```python
from build123d import *

# Parameters (mm, degrees)
SKETCH_1_W               = 30
SKETCH_1_H               = 60
EXTRUDE_1_DEPTH          = 3
SKETCH_2_W               = 26
SKETCH_2_H               = 2
EXTRUDE_3_DEPTH          = 70
SKETCH_4_R               = 5
CUT_EXTRUDE_2_DEPTH      = 21.5
CUT_EXTRUDE_3_DEPTH      = 91.58835466
CUT_EXTRUDE_3_DEPTH_BACK = 91.58835466
SKETCH_5_R               = 1.5
SKETCH_7_W               = 29.85954739
SKETCH_7_H               = 3
EXTRUDE_4_DEPTH          = 3
CUT_EXTRUDE_5_DEPTH      = 82.504601097
CUT_EXTRUDE_5_DEPTH_BACK = 82.504601097
SKETCH_8_R               = 2


with BuildPart() as part:
    # 草图1 → 凸台-拉伸1 (new body)
    with BuildSketch(Plane(origin=(0, 0, 0), x_dir=(1, 0, 0), z_dir=(0, 1, 0))):
        Rectangle(SKETCH_1_W, SKETCH_1_H)
    extrude(amount=EXTRUDE_1_DEPTH)

    # 草图2 → 凸台-拉伸3 (add)
    with BuildSketch(Plane(origin=(0, 3, 0), x_dir=(1, 0, 0), z_dir=(0, 1, 0))):
        with Locations((0, 22)):
            Rectangle(SKETCH_2_W, SKETCH_2_H)
        with Locations((0, -22)):
            Rectangle(SKETCH_2_W, SKETCH_2_H)
    extrude(amount=EXTRUDE_3_DEPTH)

    # 草图4 → 切除-拉伸2 (cut, symmetric)
    with BuildSketch(Plane.XY):
        with Locations((0, 53)):
            Circle(SKETCH_4_R)
    extrude(amount=CUT_EXTRUDE_2_DEPTH, both=True, mode=Mode.SUBTRACT)

    # 草图5 → 切除-拉伸3 (cut, two sides: drawn at the far end of the back side and taken through both)
    with BuildSketch(Plane.XY.offset(-21.5).offset(-CUT_EXTRUDE_3_DEPTH_BACK)):
        with Locations((0, 53)):
            Circle(SKETCH_5_R)
    extrude(amount=CUT_EXTRUDE_3_DEPTH + CUT_EXTRUDE_3_DEPTH_BACK, mode=Mode.SUBTRACT)

    # 草图7 → 凸台-拉伸4 (add)
    with BuildSketch(Plane.XZ):
        Polygon((-14.929773695, 33), (-14.929773695, 30), (-12, 30), (14.929773695, 30), (14.929773695, 33), align=None)
        with Locations((0, -31.5)):
            Rectangle(SKETCH_7_W, SKETCH_7_H)
    extrude(amount=-EXTRUDE_4_DEPTH)

    # 草图8 → 切除-拉伸5 (cut, two sides: drawn at the far end of the back side and taken through both)
    with BuildSketch(Plane.XZ.offset(-CUT_EXTRUDE_5_DEPTH_BACK)):
        with BuildLine():
            ThreePointArc((-8.929773695, 29), (-9.515560133, 30.414213562), (-10.929773695, 31))
            Line((-10.929773695, 31), (-10.929773695, 29))
            Line((-10.929773695, 29), (-12.929773695, 29))
            ThreePointArc((-12.929773695, 29), (-10.929773695, 27), (-8.929773695, 29))
        make_face()
        with BuildLine():
            Line((-10.929773695, 29), (-10.929773695, 31))
            ThreePointArc((-10.929773695, 31), (-12.343987258, 30.414213562), (-12.929773695, 29))
            Line((-12.929773695, 29), (-10.929773695, 29))
        make_face()
        with Locations(Location((10.929773695, 29, 0), (0, 0, 270))):
            Circle(SKETCH_8_R)
        with Locations(Location((-10.929773695, -29, 0), (0, 0, 270))):
            Circle(SKETCH_8_R)
        with Locations(Location((10.929773695, -29, 0), (0, 0, 270))):
            Circle(SKETCH_8_R)
    extrude(amount=CUT_EXTRUDE_5_DEPTH + CUT_EXTRUDE_5_DEPTH_BACK, mode=Mode.SUBTRACT)


solid = part.part
```
Can you work these out from the model? Positions are in its coordinate system, mm. A direction names the side the tool comes from. Round coordinates to 2 decimals unless told otherwise and drop trailing zeros. Order: outer loops, then holes, each group sorted by start corner. A loop starts at its lowest first (then second) coordinate and runs counter-clockwise, first axis right, second up.
(1) If we section it at B-B (x = 0): Please give me the cut outline in (y, z).
Results are:
outline: (0, -33) - (3, -33) - (3, -23) - (51.5, -23) - (51.5, -21.5) - (48, -21.5) - (48, -21) - (3, -21) - (3, 21) - (48, 21) - (48, 21.5) - (51.5, 21.5) - (51.5, 23) - (3, 23) - (3, 33) - (0, 33) - close; (54.5, -23) - (73, -23) - (73, -21) - (58, -21) - (58, -21.5) - (54.5, -21.5) - close; (54.5, 21.5) - (58, 21.5) - (58, 21) - (73, 21) - (73, 23) - (54.5, 23) - close
(2) We'd pull the mould along Z, two halves only. Please class faces 6 (the face through (0, 1, -33)), 7 (the face through (-0.325, 51.536, 22.239)), 8 (the face through (-1.2, 54.2, 21.5)): +Z half, -Z half, draft (parallel to the pull), parting line (faces both ways), or undercut.
Results are:
face 6: -Z half
face 7: draft
face 8: undercut
(3) If we section it at A-A (y = 53): Please give me the cut outline in (x, z), plus the area to 3 significant figures.
Results are:
outline: (-13, -23) - (-1.5, -23) - (-1.5, -21.5) - (-5, -21.5) - (-5, -21) - (-13, -21) - close; (-13, 21) - (-5, 21) - (-5, 21.5) - (-1.5, 21.5) - (-1.5, 23) - (-13, 23) - close; (1.5, -23) - (13, -23) - (13, -21) - (5, -21) - (5, -21.5) - (1.5, -21.5) - close; (1.5, 21.5) - (5, 21.5) - (5, 21) - (13, 21) - (13, 23) - (1.5, 23) - close
area: 85.0 mm2
(4) If we section it at C-C (z = -29): Please give me the cut outline in (x, y).
Results are:
outline: (-15, 0) - (-12.93, 0) - (-12.93, 3) - (-15, 3) - close; (-8.93, 0) - (8.93, 0) - (8.93, 3) - (-8.93, 3) - close; (12.93, 0) - (15, 0) - (15, 3) - (12.93, 3) - close
(5) I'm going to push flat-ended pins straight in: pin 1 (15 mm diameter, centred on x = 1.5, z = 1, fed in from +Y); pin 2 (3.5 mm diameter, centred on y = 1, z = 31, fed in from +X); pin 3 (5 mm diameter, centred on y = 17.5, z = -22.5, fed in from -X); pin 4 (2.5 mm diameter, centred on y = 2, z = 31.5, fed in from -X). Where does each tip first touch, or does it pass through?
Results are:
pin 1: stops at y = 3
pin 2: stops at x = 15
pin 3: stops at x = -13
pin 4: stops at x = -14.93
(6) If I drill on L1, parallel to Z at x = -0.75, y = 57.5; L2, parallel to Z at x = 5, y = 34; L3, parallel to X at y = 1, z = -29, over which ranges is the centre line in solid material (lowest first)?
Results are:
L1: z = -23 to -21.5, 21.5 to 23
L2: z = -23 to -21, 21 to 23
L3: x = -15 to -12.93, -8.93 to 8.93, 12.93 to 15
(7) On a 3-axis mill with a long thin cutter (end or side, diameter ignored), from which of +Z, -Z, +X, -X, +Y, -Y can I reach the whole of each face in a straight line? I mean faces 1 (the face through (-14.93, 1, 32)), 2 (the face through (-0.651, 57.957, 21.254)), 3 (the face through (0, 38, -23)), 4 (the face through (0, 38, -21)), 5 (the face through (-13, 38, 22)). Say none if no direction works.
Results are:
face 1: +Z, -X, +Y, -Y
face 2: none
face 3: -Z, +X, -X, +Y
face 4: +X, -X, +Y
face 5: +Z, -Z, -X, +Y
(8) If we section it at D-D (y = 7.5): Please give me the cut outline in (x, z), plus the area to 3 significant figures.
Results are:
outline: (-13, -23) - (13, -23) - (13, -21) - (-13, -21) - close; (-13, 21) - (13, 21) - (13, 23) - (-13, 23) - close
area: 104 mm2
